Geometry: final body of the model. Coordinates: model frame, mm. Face numbers are marked on the shaded views. Give positions to 0.01 mm unless a question says otherwise; leave off trailing zeros. Loops run counter-clockwise (first coordinate to the right, second up) from the corner with the lowest first, then second, coordinate; pieces in that order, holes last.
from build123d import *

# Parameters (mm, degrees)
SKETCH1_W           = 500
SKETCH1_H           = 185
BOSS_EXTRUDE1_DEPTH = 3
SKETCH2_W           = 45.28
SKETCH2_H           = 25.85
CUT_EXTRUDE1_DEPTH  = 3


with BuildPart() as part:
    # Sketch1 → Boss-Extrude1 (new body)
    with BuildSketch(Plane(origin=(0, 0, 0), x_dir=(1, 0, 0), z_dir=(0, 1, 0))):
        with Locations((0, -2.5)):
            Rectangle(SKETCH1_W, SKETCH1_H)
    extrude(amount=BOSS_EXTRUDE1_DEPTH)

    # Sketch2 → Cut-Extrude1 (cut)
    with BuildSketch(Plane(origin=(0, 3, 0), x_dir=(1, 0, 0), z_dir=(0, 1, 0))):
        with Locations((-42.64, 57.075)):
            Rectangle(SKETCH2_W, SKETCH2_H)
        with Locations((42.64, 57.075)):
            Rectangle(SKETCH2_W, SKETCH2_H)
    extrude(amount=-CUT_EXTRUDE1_DEPTH, mode=Mode.SUBTRACT)


solid = part.part
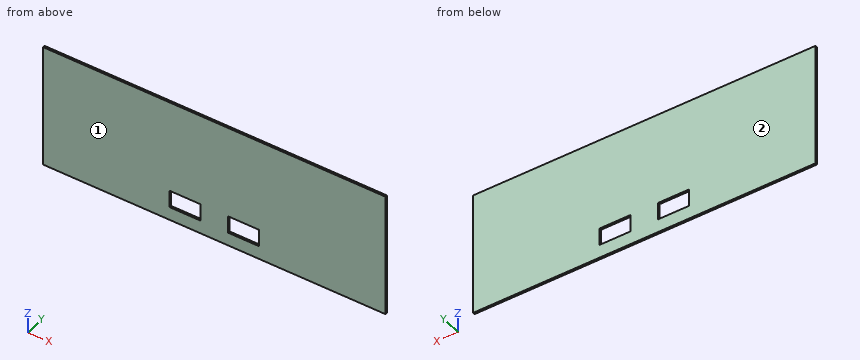
Item 1: Draft query along Y for the marked faces 1 and 2. Return one class per face: +Y half, -Y half, draft (parallel to the pull), parting line (faces both ways), or undercut.
Values follow:
face 1: -Y half
face 2: +Y half
Item 2: Ray query, probe 1 along X at (y, z) = (0.8, -64); probe 2 along Z at (x, y) = (-34.5, 0.95). Return the intervals inside material, ascending.
Values follow:
probe 1: x = -250 to -65.28, -20 to 20, 65.28 to 250
probe 2: z = -90 to -70, -44.15 to 95
Item 3: Section query A-A on x = -39.5. Return loops of the section in (y, z).
Values follow:
outline: (0, -90) - (3, -90) - (3, -70) - (0, -70) - close; (0, -44.15) - (3, -44.15) - (3, 95) - (0, 95) - close
Item 4: Section query B-B on y = 1.6. Return loops of the section in (x, z), plus the area to 3 significant figures.
Values follow:
outline: (-250, -90) - (250, -90) - (250, 95) - (-250, 95) - close; hole (-65.28, -70) - (-20, -70) - (-20, -44.15) - (-65.28, -44.15) - close; hole (20, -70) - (65.28, -70) - (65.28, -44.15) - (20, -44.15) - close
area: 90,200 mm2
